For this review, take the finished solid that the model builds, in its own axes (mm). Face numbers are marked on the shaded views. A direction names the side the tool comes from. Round coordinates to 2 decimals unless told otherwise and drop trailing zeros. Write each loop counter-clockwise with the first axis right and the second up, starting at its lowest first coordinate (ties: lowest second). Pieces come first, ordered by that corner, then holes. Notation, with made-up numbers: (-13, -15.75) - (10, -15.75) arc R17 ccw to (10, -9.75) - close; hole circle Ø3 at (71, 64). An arc over 180 degrees is marked (long way). One line per item, written item: value. Start each with the question number.
Q1. Clearance check with flat-ended pins moving along their axes: pin 1 Ø3 at (x, z) = (6, -54.5) entering from +Y; pin 2 Ø19.5 at (x, z) = (5.42, -8.17) entering from -Y. State where each tip first meets the part, or that it passes through.
Q2. Add section A-A on x = 28.5. Write out the cut boundary in (y, z).
Q3. Mouldability with a two-part tool opening along X and no side actions: class the marked faces 3, 4 and 5 as +X half, -X half, draft (parallel to the pull), parting line (faces both ways), or undercut.
Q4. For probe 1 along X at (y, z) = (15, -27); probe 2 along X at (y, z) = (55.5, -38); probe 3 along X at (y, z) = (15, 14), list the stretches that pass through material, from the lowest coordinate up.
Q5. Tool access review of the marked faces 1 and 2: name each direction out of +Z, -Z, +X, -X, +Y, -Y from which nothing blocks a thin tool from reaching the whole face with its end or side.
Q6. Add section B-B on y = 37.5. Write out the cut boundary in (x, z), and give its area (3 significant figures).
Q7. Add section C-C on z = -23. Write out the cut boundary in (x, y), and give its area (3 significant figures).
Autodesk Inventor part; units mm, degrees
ref_plane "YZ Plane" through (0, 0, 0) normal (1, 0, 0) x (0, 1, 0)
ref_plane "XZ Plane" through (0, 0, 0) normal (0, 1, 0) x (-1, 0, 0)
ref_plane "XY Plane" through (0, 0, 0) normal (0, 0, 1) x (1, 0, 0)
sketch "스케치1" plane through (0, 0, 0) normal (0, 1, 0) x (-1, 0, 0)
  line L0 (60, 80) -> (-60, 80)
  line L1 (-60, 80) -> (-60, -80)
  line L2 (-60, -80) -> (60, -80)
  line L3 (60, -80) -> (60, 80)
  line L4 (60, 80) -> (-60, -80) construction
  line L5 (-60, 80) -> (60, -80) construction
  point P0 (0, 0)
  dimension "d0" = 120
  dimension "d1" = 160
extrude "돌출1" add sketch "스케치1" along normal blind 60
sketch "스케치2" plane through (0, 60, 0) normal (0, 1, 0) x (1, 0, 0)
  line L0 (60, -80) -> (60, 80)
  line L1 (60, 80) -> (-60, 80)
  line L2 (55, 102.1646) -> (-55, 102.1646)
  line L3 (-55, 102.1646) -> (-55, -89.711)
  line L4 (-55, -89.711) -> (55, -89.711)
  line L5 (55, -89.711) -> (55, 102.1646)
  line L6 (-60, 80) -> (-60, -80)
  point P0 (0, 0)
  point P1 (55, 80)
  point P2 (-55, 80)
  dimension "d6" = 5
  dimension "d7" = 5
extrude "돌출2" cut sketch "스케치2" against normal blind 40 contours L5 L4 L3 L1
sketch "스케치12" plane through (60, 0, -80) normal (0, 0, -1) x (-1, 0, 0)
  line L0 (-34.8463, 10) -> (156.2634, 10)
  line L1 (156.2634, 10) -> (156.2634, -36.9465)
  line L2 (156.2634, -36.9465) -> (-34.8463, -36.9465)
  line L3 (-34.8463, -36.9465) -> (-34.8463, 10)
  line L4 (0, 0) -> (120, 0)
  point P0 (60, 0)
  dimension "d85" = 10
extrude "돌출10" cut sketch "스케치12" against normal through all
sketch "스케치13" plane through (-55, 20, 80) normal (0, 0, 1) x (1, 0, 0)
  line L0 (0, 40) -> (0, 0)
  line L1 (0, 0) -> (110, 0)
  line L2 (0, 40) -> (110, 40)
  line L3 (110, 40) -> (110, 0)
  line L4 (110, 0) -> (0, 0)
  line L5 (0, 0) -> (0, 40)
  point P0 (55, -20)
extrude "돌출11" add sketch "스케치13" against normal blind 5
sketch "스케치14" plane through (55, 20, -80) normal (0, 0, -1) x (-1, 0, 0)
  line L0 (0, 0) -> (0, 40)
  line L1 (110, 0) -> (0, 0)
  line L2 (0, 40) -> (110, 40)
  line L3 (110, 40) -> (110, 0)
  line L4 (110, 0) -> (0, 0)
  line L5 (0, 0) -> (0, 40)
  point P0 (55, -20)
extrude "돌출12" add sketch "스케치14" against normal blind 5
sketch "스케치15" plane through (60, 60, -80) normal (0, 0, -1) x (-1, 0, 0)
  point P0 (60, -60)
sketch "스케치16" plane through (60, 60, -80) normal (0, 0, -1) x (-1, 0, 0)
  point P0 (60, -60)
sketch "스케치17" plane through (0, 20, 0) normal (0, 1, 0) x (1, 0, 0)
  line L0 (7, 27) -> (45, 27)
  line L1 (45, 27) -> (45, 65)
  line L2 (45, 65) -> (7, 65)
  line L3 (7, 65) -> (7, 27)
  line L4 (55, 75) -> (55, -75)
  line L5 (55, 75) -> (-55, 75)
  circle A0 centre (7, 27) radius 1.6
  circle A1 centre (7, 65) radius 1.6
  circle A2 centre (45, 65) radius 1.6
  circle A3 centre (45, 27) radius 1.6
  line L6 (-47.9371, 14.7215) -> (-7.9371, 14.7215)
  line L7 (-7.9371, 14.7215) -> (-7.9371, 64.7215)
  line L8 (-7.9371, 64.7215) -> (-47.9371, 64.7215)
  line L9 (-47.9371, 64.7215) -> (-47.9371, 14.7215)
  point P0 (0, 0)
  dimension "d92" = 38
  dimension "d93" = 38
  dimension "d95" = 10
  dimension "d96" = 10
  dimension "d97" = 3.2
  dimension "d98" = 3.2
  dimension "d99" = 3.2
  dimension "d100" = 3.2
  dimension "d113" = 40
  dimension "d114" = 50
extrude "돌출13" cut sketch "스케치17" against normal through all contours L3 A0 L0 | L0 A0 L3 | A3 L1 L0 | L0 L1 A3 | A1 L2 L3 | L3 L2 A1 | A2 L2 L1 | L1 L2 A2
sketch "스케치21" plane through (0, 20, 0) normal (0, 1, 0) x (1, 0, 0)
  circle A0 centre (5.4243, 8.1678) radius 7.5
  line L0 (-49.3888, 17.2731) -> (-9.3888, 17.2731)
  line L1 (-9.3888, 17.2731) -> (-9.3888, 67.2731)
  line L2 (-9.3888, 67.2731) -> (-49.3888, 67.2731)
  line L3 (-49.3888, 67.2731) -> (-49.3888, 17.2731)
  point P0 (0, 0)
  dimension "d117" = 15
  dimension "d118" = 50
  dimension "d119" = 40
extrude "돌출15" cut sketch "스케치21" against normal through all contours A0
sketch "스케치23" plane through (0, 20, 0) normal (0, 1, 0) x (1, 0, 0)
  line L0 (-48.6, -65) -> (20, -65)
  line L1 (20, -65) -> (20, -11.6)
  line L2 (20, -11.6) -> (-48.6, -11.6)
  line L3 (-48.6, -11.6) -> (-48.6, -65)
  line L4 (55, 75) -> (55, -75)
  line L5 (-55, -75) -> (55, -75)
  circle A0 centre (4.7, -62.45) radius 1.6
  circle A1 centre (6.03, -14.15) radius 1.6
  circle A2 centre (-46.05, -47.16) radius 1.6
  circle A3 centre (-46.05, -19.23) radius 1.6
  point P0 (0, 0)
  dimension "d123" = 68.6
  dimension "d124" = 53.4
  dimension "d125" = 35
  dimension "d126" = 10
  dimension "d127" = 3.2
  dimension "d128" = 15.3
  dimension "d129" = 2.55
  dimension "d130" = 3.2
  dimension "d131" = 13.97
  dimension "d132" = 2.55
  dimension "d133" = 3.2
  dimension "d134" = 35.56
  dimension "d135" = 3.2
  dimension "d136" = 2.55
  dimension "d137" = 2.55
  dimension "d138" = 7.63
extrude "돌출16" cut sketch "스케치23" against normal through all contours A0 | A1 | A2 | A3
properties part number "본체 회전"
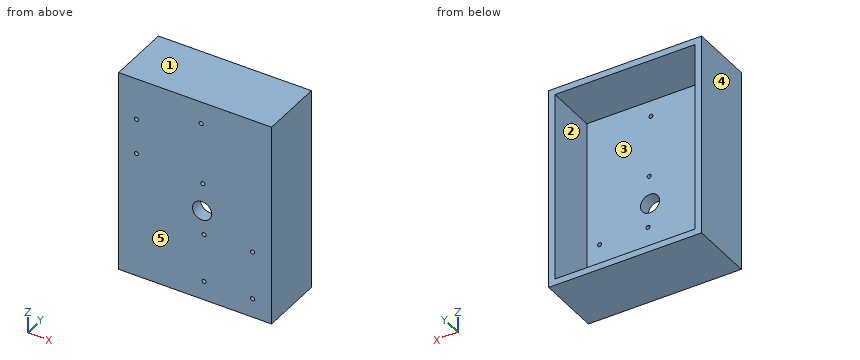
Result set:
1. pin 1: stops at y = 20
1. pin 2: stops at y = 10
2. outline: (10, -80) - (60, -80) - (60, -75) - (20, -75) - (20, 75) - (60, 75) - (60, 80) - (10, 80) - close
3. face 3: undercut
3. face 4: -X half
3. face 5: draft
4. probe 1: x = -60 to 5.4, 8.6 to 43.4, 46.6 to 60
4. probe 2: x = -60 to -55, 55 to 60
4. probe 3: x = -60 to 4.44, 7.62 to 60
5. face 1: +Z, +X, -X, +Y, -Y
5. face 2: +Y
6. outline: (-60, -80) - (60, -80) - (60, 80) - (-60, 80) - close; hole (-55, -75) - (55, -75) - (55, 75) - (-55, 75) - close
6. area: 2,700 mm^2
7. outline: (-60, 10) - (60, 10) - (60, 60) - (55, 60) - (55, 20) - (-55, 20) - (-55, 60) - (-60, 60) - close
7. area: 1,600 mm^2
